from build123d import *

# Parameters (mm, degrees)
BOSS_EXTRUDE1_DEPTH = 70.26


with BuildPart() as part:
    # Loft13: read off the stored shape, not the designer's step
    # Loft13: loft between two sections, ruled curve by curve
    loft13_from = [
        Edge.make_bspline([(-100.000171146, 11.035604797, 30), (-99.166809288, 10.690415013, 30), (-98.33344743, 10.345225229, 30), (-96.666723715, 9.654845662, 30), (-95.833361858, 9.309655878, 30), (-95, 8.964466094, 30)], [0, 0, 0, 0, 0.5, 0.5, 1, 1, 1, 1], 3),
        Edge.make_bspline([(-95, 8.964466094, 30), (-94.590223449, 9.374207863, 30), (-94.180446899, 9.783949632, 30), (-93.360893797, 10.603433171, 30), (-92.951117247, 11.01317494, 30), (-92.541340696, 11.422916709, 30)], [0, 0, 0, 0, 0.5, 0.5, 1, 1, 1, 1], 3),
        Edge.make_bspline([(-76.034367882, 34.999373863, 30), (-80.028668426, 31.005412352, 30), (-84.02296897, 27.011450841, 30), (-92.011570058, 19.023527819, 30), (-96.005870602, 15.029566308, 30), (-100.000171146, 11.035604797, 30)], [0, 0, 0, 0, 0.5, 0.5, 1, 1, 1, 1], 3),
        Edge.make_bspline([(-92.541340696, 11.422916709, 30), (-89.444897324, 14.519097257, 30), (-86.348453952, 17.615277806, 30), (-80.155567208, 23.807638903, 30), (-77.059123835, 26.903819451, 30), (-73.962680463, 30, 30)], [0, 0, 0, 0, 0.5, 0.5, 1, 1, 1, 1], 3),
        Edge.make_bspline([(-73.962680463, 30, 30), (-49.307680463, 30, 30), (-24.652680463, 30, 30), (24.657319537, 30, 30), (49.312319537, 30, 30), (73.967319537, 30, 30)], [0, 0, 0, 0, 0.5, 0.5, 1, 1, 1, 1], 3),
        Edge.make_bspline([(73.967319537, 30, 30), (77.473093055, 26.493928889, 30), (80.978866573, 22.987857778, 30), (87.99041361, 15.975715557, 30), (91.496187128, 12.469644446, 30), (95.001960646, 8.963573335, 30)], [0, 0, 0, 0, 0.5, 0.5, 1, 1, 1, 1], 3),
        Edge.make_bspline([(95.001960646, 8.963573335, 30), (95.834992025, 9.30862623, 30), (96.668023403, 9.653679125, 30), (98.33408616, 10.343784915, 30), (99.167117539, 10.68883781, 30), (100.000148917, 11.033890705, 30)], [0, 0, 0, 0, 0.5, 0.5, 1, 1, 1, 1], 3),
        Edge.make_bspline([(100.000148917, 11.033890705, 30), (96.006240753, 15.028137898, 30), (92.012332588, 19.022385091, 30), (84.024516259, 27.010879477, 30), (80.030608095, 31.00512667, 30), (76.03669993, 34.999373863, 30)], [0, 0, 0, 0, 0.5, 0.5, 1, 1, 1, 1], 3),
        Edge.make_bspline([(76.03669993, 34.999373863, 30), (63.364110946, 34.999373863, 30), (50.691521962, 34.999373863, 30), (25.346343993, 34.999373863, 30), (12.673755009, 34.999373863, 30), (0.001166024, 34.999373863, 30)], [0, 0, 0, 0, 0.5, 0.5, 1, 1, 1, 1], 3),
        Edge.make_bspline([(0.001166024, 34.999373863, 30), (-12.67142296, 34.999373863, 30), (-25.344011944, 34.999373863, 30), (-50.689189913, 34.999373863, 30), (-63.361778897, 34.999373863, 30), (-76.034367882, 34.999373863, 30)], [0, 0, 0, 0, 0.5, 0.5, 1, 1, 1, 1], 3),
    ]
    loft13_to = [
        Edge.make_bspline([(-100, 0, 57.735026919), (-98.821488698, 0, 57.735026919), (-97.642977396, 0, 57.735026919), (-95.285954792, 0, 57.735026919), (-94.10744349, 0, 57.735026919), (-92.928932188, 0, 57.735026919)], [0, 0, 0, 0, 0.5, 0.5, 1, 1, 1, 1], 3),
        Edge.make_bspline([(-92.928932188, 0, 57.735026919), (-86.631916235, 0, 64.032042873), (-80.334900281, 0, 70.329058826), (-67.740868375, 0, 82.923090733), (-61.443852421, 0, 89.220106686), (-55.146836468, 0, 95.517122639)], [0, 0, 0, 0, 0.5, 0.5, 1, 1, 1, 1], 3),
        Edge.make_bspline([(-57.735026919, 0, 100), (-64.779189099, 0, 92.95583782), (-71.823351279, 0, 85.91167564), (-85.91167564, 0, 71.82335128), (-92.95583782, 0, 64.7791891), (-100, 0, 57.735026919)], [0, 0, 0, 0, 0.5, 0.5, 1, 1, 1, 1], 3),
        Edge.make_bspline([(-55.146836468, 0, 95.517122639), (-45.955697057, 0, 97.979881022), (-36.764557645, 0, 100.442639405), (-18.382278823, 0, 105.368156171), (-9.191139411, 0, 107.830914553), (0, 0, 110.293672936)], [0, 0, 0, 0, 0.5, 0.5, 1, 1, 1, 1], 3),
        Edge.make_bspline([(0, 0, 110.293672936), (9.191139411, 0, 107.830914553), (18.382278823, 0, 105.368156171), (36.764557645, 0, 100.442639405), (45.955697057, 0, 97.979881022), (55.146836468, 0, 95.517122639)], [0, 0, 0, 0, 0.5, 0.5, 1, 1, 1, 1], 3),
        Edge.make_bspline([(55.146836468, 0, 95.517122639), (61.443852421, 0, 89.220106686), (67.740868375, 0, 82.923090733), (80.334900281, 0, 70.329058826), (86.631916235, 0, 64.032042873), (92.928932188, 0, 57.735026919)], [0, 0, 0, 0, 0.5, 0.5, 1, 1, 1, 1], 3),
        Edge.make_bspline([(92.928932188, 0, 57.735026919), (94.10744349, 0, 57.735026919), (95.285954792, 0, 57.735026919), (97.642977396, 0, 57.735026919), (98.821488698, 0, 57.735026919), (100, 0, 57.735026919)], [0, 0, 0, 0, 0.5, 0.5, 1, 1, 1, 1], 3),
        Edge.make_bspline([(100, 0, 57.735026919), (92.95583782, 0, 64.7791891), (85.91167564, 0, 71.82335128), (71.823351279, 0, 85.91167564), (64.779189099, 0, 92.95583782), (57.735026919, 0, 100)], [0, 0, 0, 0, 0.5, 0.5, 1, 1, 1, 1], 3),
        Edge.make_bspline([(57.735026919, 0, 100), (48.112522433, 0, 102.578342307), (38.490017946, 0, 105.156684613), (19.245008973, 0, 110.313369226), (9.622504487, 0, 112.891711532), (0, 0, 115.470053838)], [0, 0, 0, 0, 0.5, 0.5, 1, 1, 1, 1], 3),
        Edge.make_bspline([(0, 0, 115.470053838), (-9.622504487, 0, 112.891711532), (-19.245008973, 0, 110.313369226), (-38.490017946, 0, 105.156684613), (-48.112522433, 0, 102.578342307), (-57.735026919, 0, 100)], [0, 0, 0, 0, 0.5, 0.5, 1, 1, 1, 1], 3),
    ]
    loft13 = Solid(Shell([*[Face.make_surface_from_curves(loft13_from[k], loft13_to[k]) for k in range(10)], Face(Wire(loft13_from)), Face(Wire(loft13_to))]))
    add(loft13)

    # Sketch9 → Boss-Extrude1 (add)
    with BuildSketch(Plane.XY.offset(30)):
        Polygon((100.000148917, 11.033890705), (95.001960646, 8.963573335), (73.967319537, 30), (-73.962680463, 30), (-95, 8.964466094), (-100.000171146, 11.035604797), (-76.034367882, 34.999373863), (76.03669993, 34.999373863), align=None)
    extrude(amount=-BOSS_EXTRUDE1_DEPTH)


solid = part.part
Design review of the part built by this model. Coordinates are the model's own, in mm. A direction names the side the tool comes from. Round coordinates to 2 decimals unless told otherwise and drop trailing zeros. Write each loop counter-clockwise with the first axis right and the second up, starting at its lowest first coordinate (ties: lowest second). Pieces come first, ordered by that corner, then holes. Notation, with made-up numbers: (74.25, 81) -> (108.25, 81) arc R29 ccw to (108.25, 102) -> close; hole circle Ø7 at (32.25, 28). An arc over 180 degrees is marked (long way). One line per question, with ' | ' between items.
(1) Machinability: for faces 5 (the flat face through (-88.185, 22.85, -4.638)), 6 (the flat face through (-97.5, 10, -4.6)), 7 (the flat face through (-84.334, 19.629, -4.638)), which of the approach directions +Z, -Z, +X, -X, +Y, -Y give a long, thin tool a straight path to every point of the face, cutting with its end or side? Answer none if there is none.
Result sheet:
face 5: +Z, -Z, -X, +Y | face 6: -Z, -X, -Y | face 7: -Z, -Y
(2) Take a section at A-A, the plane z = 18. State the section outline as (x, y) points.
Result sheet:
outline: (-100, 11.04) -> (-95, 8.96) -> (-73.96, 30) -> (73.97, 30) -> (95, 8.96) -> (100, 11.03) -> (76.04, 35) -> (-76.03, 35) -> close
(3) Wall thickness on line 1 (Y direction, x = 1.5, z = 13); line 2 (X direction, y = 3, z = 77.5); line 3 (Y direction, x = 25.5, z = 98): over which ranges is each line inside the solid? List them lowest first. Write a range as [from, to].
Result sheet:
line 1: [30, 35] | line 2: [-75.29, -65.75], [68.06, 75.29] | line 3: [2.04, 4.84]
(4) Draft analysis for pull direction X (two halves, no side actions). For faces 1 (the flat face through (-1, 34.999, -5)), 2 (the flat face through (84.632, 19.335, -4.638)), 3 (the flat face through (97.5, 10, -4.6)), 4 (the flat face through (1, 30, -5)), state which applies: released by +X, released by -X, zero draft, split by the parting line, or undercut.
Result sheet:
face 1: zero draft | face 2: undercut | face 3: released by +X | face 4: undercut
(5) Insertion check: P1, Ø21, axis at x = 16.5, z = -9, coming from the -Y side; P2, Ø8, axis at x = -17, z = 36.5, coming from the -Y side; P3, Ø12, axis at x = 79.5, z = 52.5, coming from the -Y side. Each pin has a flat end and moves straight along its axis. Give the tip position at first contact, or say it passes through.
Result sheet:
P1: y = 30 | P2: y = 25.81 | P3: y = 4.85
